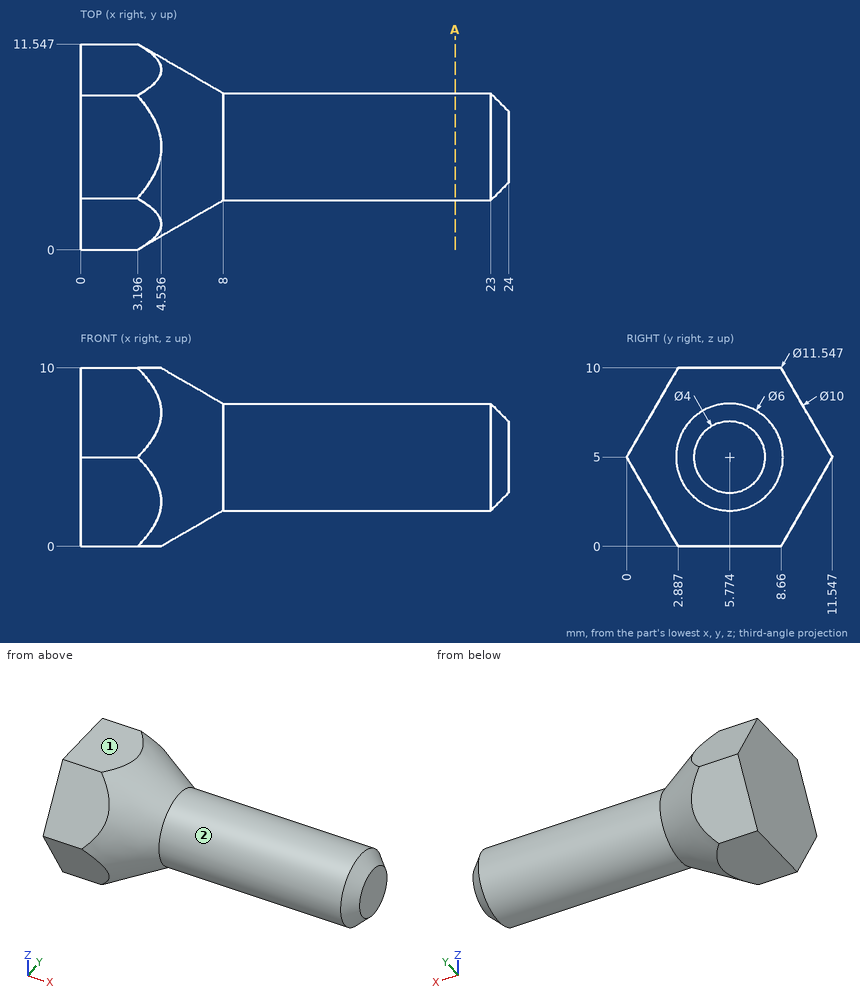
Print and shaded views of the part. All mm, measured from the part's lowest x, y and z. A direction names the side the tool comes from. Give positions to 0.01 mm unless a question says otherwise; leave off trailing zeros. Loops run counter-clockwise (first coordinate to the right, second up) from the corner with the lowest first, then second, coordinate; pieces in that order, holes last. Notation, with made-up numbers: (3.25, 8.25) -> (40.25, 8.25) arc R22 ccw to (40.25, 37.25) -> close; hole circle Ø5 at (61.5, 10.5). An arc over 180 degrees is marked (long way). Use a Markdown table: item, result.
1. Slice it at A-A (x = 21). List the corners of the cut face in (y, z).
Check result:
| item | result |
|---|---|
| outline | circle Ø6 at (5.77, 5) |
2. Which spindle directions (+Z, -Z, +X, -X, +Y, -Y) get a long thin tool onto all of the face, cutting with end or side? Do the marked faces 1 and 2. Say none if no direction does.
Check result:
| item | result |
|---|---|
| face 1 | +Z, +X, -X, +Y, -Y |
| face 2 | +X |
3. Wall check: L1, parallel to X at y = 6.5, z = 1 (1 decimal); L2, parallel to Y at x = 18.75, z = 2.5 (1 decimal); L3, parallel to X at y = 1, z = 5.25 (1 decimal). Give the ranges that are in metal, low to high. Write a range as [from, to].
Check result:
| item | result |
|---|---|
| L1 | x = [0, 6.2] |
| L2 | y = [4.1, 7.4] |
| L3 | x = [0, 4.9] |
4. Flat gauge pins, fed straight in: pin 1 (1.5 mm diameter, centred on x = 3, y = 10, fed in from -Z); pin 2 (6 mm diameter, centred on x = 15.5, y = 4, fed in from +Z); pin 3 (1 mm diameter, centred on x = 3.5, z = 2, fed in from -Y). Where does each tip first touch, or does it go through?
Check result:
| item | result |
|---|---|
| pin 1 | stops at z = 1.02 |
| pin 2 | stops at z = 8 |
| pin 3 | stops at y = 1.44 |
